Read the model definition and answer for the solid it produces. Units are mm, in the model's axes. A direction names the side the tool comes from. Give positions to 0.01 mm unless a question says otherwise; leave off trailing zeros. Write each loop counter-clockwise with the first axis right and the second up, starting at its lowest first coordinate (ties: lowest second). Pieces come first, ordered by that corner, then holes. Notation, with made-up numbers: (83, -40) -> (123, -40) arc R22 ccw to (123, -23) -> close; hole circle Ø8 at (-8, -23.5). An arc over 180 degrees is marked (long way). Answer as CSV lines item,"result". Start each with the question number.
1. The part is cut by section D-D, the plane x = 23.5. Determine the outline of the cut face in (y, z).
2. Given pin 1 (2 mm diameter, centred on x = 5.01, y = 39.36, fed in from +Z); pin 2 (5.5 mm diameter, centred on x = 27.67, z = -14.3, fed in from +Y); pin 3 (1.5 mm diameter, centred on x = 18.5, y = 15, fed in from +Z); pin 4 (4 mm diameter, centred on x = 16.5, z = -26.5, fed in from -Y), each flat-ended and moving along its own axis, determine where each tip first touches the part or whether it passes through.
3. The part is cut by section A-A, the plane y = 7.5. Determine the outline of the cut face in (x, z), and give its area (3 significant figures).
4. Find the intervals of material crossed by line 1 (X direction, y = 8, z = -14.3); line 2 (Y direction, x = 28.5, z = -11.5); line 3 (Z direction, x = 28.5, y = 30), in increasing order.
5. The part is cut by section C-C, the plane z = -30. Determine the outline of the cut face in (x, y), and give its area (3 significant figures).
6. The part is cut by section B-B, the plane y = 18. Determine the outline of the cut face in (x, z).
7. For a pull along Z with two mould halves and no side action, classify faces 4 (the flat face through (17, 2.04, -10)), 5 (the cylindrical face through (28.939, 17.557, -31.262)), 6 (the flat face through (17, 23, -34)) as pulls with the +Z half, pulls with the -Z half, needs draft (parallel to the pull), parting line crosses it, or undercut.
8. A tool of negligible diameter and unlimited length cuts with its end or side. For faces 1 (the cylindrical face through (23.36, 7.11, -20.67)), 2 (the flat face through (24, 12.04, -21)), 3 (the cylindrical face through (28.1, 37.85, -31.26)), from which of +Z, -Z, +X, -X, +Y, -Y can it reach the whole face along a straight path? Write none if from no direction.
from build123d import *

# Parameters (mm, degrees)
SKETCH1_W           = 34
SKETCH1_H           = 34
BOSS_EXTRUDE1_DEPTH = 12.04
SKETCH2_W           = 34
SKETCH2_H           = 5.4
BOSS_EXTRUDE2_DEPTH = 34
SKETCH3_R           = 9
CUT_EXTRUDE1_DEPTH  = 10
SKETCH4_R           = 1.7
SKETCH4_R_2         = 1.700000029
CUT_EXTRUDE2_DEPTH  = 59.889727457
SKETCH6_R           = 3
CUT_EXTRUDE3_DEPTH  = 66.176682947
SKETCH7_R           = 1.7
CUT_EXTRUDE4_DEPTH  = 64.981572347


with BuildPart() as part:
    # Sketch1 → Boss-Extrude1 (new body)
    with BuildSketch(Plane(origin=(0, 0, 0), x_dir=(1, 0, 0), z_dir=(0, 1, 0))):
        with Locations((17, 17)):
            Rectangle(SKETCH1_W, SKETCH1_H)
    extrude(amount=BOSS_EXTRUDE1_DEPTH)

    # Sketch2 → Boss-Extrude2 (add)
    with BuildSketch(Plane(origin=(0, 12.04, 0), x_dir=(1, 0, 0), z_dir=(0, 1, 0))):
        with Locations((17, 31.3)):
            Rectangle(SKETCH2_W, SKETCH2_H)
    extrude(amount=BOSS_EXTRUDE2_DEPTH)

    # Sketch3 → Cut-Extrude1 (cut)
    with BuildSketch(Plane(origin=(0, 12.04, 0), x_dir=(1, 0, 0), z_dir=(0, 1, 0))):
        with Locations(Location((17, 14.3, 0), (0, 0, 270))):
            Circle(SKETCH3_R)
    extrude(amount=-CUT_EXTRUDE1_DEPTH, mode=Mode.SUBTRACT)

    # Sketch4 → Cut-Extrude2 (cut, through all)
    with BuildSketch(Plane(origin=(0, 12.04, 0), x_dir=(1, 0, 0), z_dir=(0, 1, 0))):
        with Locations(Location((6.33358771, 14.3, 0), (0, 0, 270))):
            Circle(SKETCH4_R)
        with Locations(Location((27.668868507, 14.3, 0), (0, 0, 270))):
            Circle(SKETCH4_R_2)
        with Locations(Location((17, 3.600864666, 0), (0, 0, 270))):
            Circle(SKETCH4_R)
        with Locations(Location((17, 24.997428292, 0), (0, 0, 270))):
            Circle(SKETCH4_R)
    extrude(amount=-CUT_EXTRUDE2_DEPTH, mode=Mode.SUBTRACT)

    # Sketch6 → Cut-Extrude3 (cut, through all)
    with BuildSketch(Plane(origin=(0, 2.04, 0), x_dir=(1, 0, 0), z_dir=(0, 1, 0))):
        with Locations(Location((17, 14.3, 0), (0, 0, 270))):
            Circle(SKETCH6_R)
    extrude(amount=-CUT_EXTRUDE3_DEPTH, mode=Mode.SUBTRACT)

    # Sketch7 → Cut-Extrude4 (cut, through all)
    with BuildSketch(Plane.XY.offset(-28.6)):
        with Locations((5.006682724, 39.357086706)):
            Circle(SKETCH7_R)
        with Locations((27.317086706, 39.357086706)):
            Circle(SKETCH7_R)
        with Locations((5.006682724, 17.046682724)):
            Circle(SKETCH7_R)
        with Locations((27.317086706, 17.046682724)):
            Circle(SKETCH7_R)
    extrude(amount=-CUT_EXTRUDE4_DEPTH, mode=Mode.SUBTRACT)


solid = part.part
Results found:
1,outline,"(0, -34) -> (46.04, -34) -> (46.04, -28.6) -> (12.04, -28.6) -> (12.04, -20.52) -> (2.04, -20.52) -> (2.04, -8.08) -> (12.04, -8.08) -> (12.04, 0) -> (0, 0) -> close"
2,pin 1,"passes through"
2,pin 2,"stops at y = 12.04"
2,pin 3,"stops at z = -28.6"
2,pin 4,"stops at y = 0"
3,outline,"(0, -34) -> (34, -34) -> (34, 0) -> (0, 0) -> close; hole (8.01, -14.61) arc R9 ccw to (16.91, -23.3) arc R1.7 ccw (long way) to (17.09, -23.3) arc R9 ccw to (26, -14.6) arc R1.7 ccw (long way) to (26, -14) arc R9 ccw to (17.05, -5.3) arc R1.7 ccw (long way) to (16.95, -5.3) arc R9 ccw to (8.01, -13.99) arc R1.7 ccw (long way) to start"
3,area,"865 mm²"
4,line 1,"x = 0 to 4.63, 29.37 to 34"
4,line 2,"y = 0 to 12.04"
4,line 3,"z = -34 to -28.6"
5,outline,"(0, 0) -> (34, 0) -> (34, 46.04) -> (0, 46.04) -> close; hole circle Ø3.4 at (5.01, 17.05); hole circle Ø3.4 at (5.01, 39.36); hole circle Ø3.4 at (27.32, 17.05); hole circle Ø3.4 at (27.32, 39.36)"
5,area,"1,530 mm²"
6,outline,"(0, -34) -> (3.6, -34) -> (3.6, -28.6) -> (0, -28.6) -> close; (6.41, -34) -> (25.91, -34) -> (25.91, -28.6) -> (6.41, -28.6) -> close; (28.72, -34) -> (34, -34) -> (34, -28.6) -> (28.72, -28.6) -> close"
7,face 4,"undercut"
7,face 5,"needs draft"
7,face 6,"pulls with the -Z half"
8,face 1,"+Y"
8,face 2,"+Z, +X, -X, +Y"
8,face 3,"+Z, -Z"
